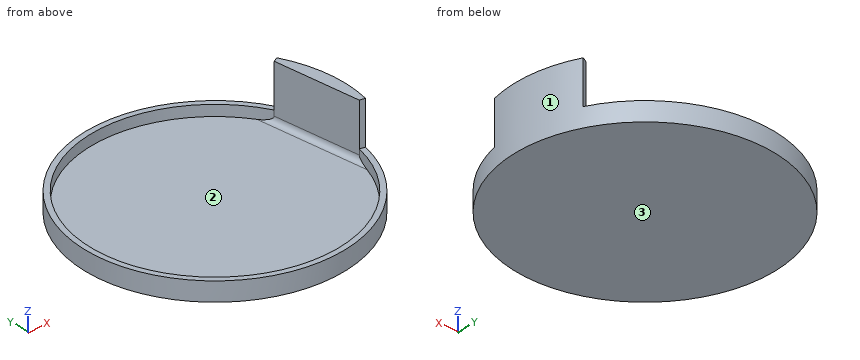
```python
from build123d import *

# Parameters (mm, degrees)
SKETCH1_R           = 48
BOSS_EXTRUDE1_DEPTH = 3
SKETCH2_R           = 48
SKETCH2_R_2         = 46
BOSS_EXTRUDE2_DEPTH = 4
BOSS_EXTRUDE3_DEPTH = 20
FILLET1_R           = 2


# Read off the part's stored shape, not the designer's step: Boss-Extrude3
with BuildPart() as part:
    # Sketch1 → Boss-Extrude1 (new body)
    with BuildSketch(Plane(origin=(0, 0, 0), x_dir=(0, 1, 0), z_dir=(0, 0, 1))):
        with Locations(Location((0, 0, 0), (0, 0, 270))):
            Circle(SKETCH1_R)
    extrude(amount=BOSS_EXTRUDE1_DEPTH)

    # Sketch2 → Boss-Extrude2 (add)
    with BuildSketch(Plane.XY.offset(3)):
        Circle(SKETCH2_R)
        Circle(SKETCH2_R_2, mode=Mode.SUBTRACT)
    extrude(amount=BOSS_EXTRUDE2_DEPTH)

    # Boss-Extrude3 outline → Boss-Extrude3 (add)
    with BuildSketch(Plane.XY.offset(3)):
        with BuildLine():
            ThreePointArc((46.862031324, -10.389899911), (47.589460087, 6.264446393), (42.576897618, 22.163208008))
            Line((42.576897618, 22.163208008), (40.802860217, 21.239741008))
            Line((40.802860217, 21.239741008), (44.909446686, -9.956987415))
            Line((44.909446686, -9.956987415), (46.862031324, -10.389899911))
        make_face()
    extrude(amount=BOSS_EXTRUDE3_DEPTH)

    # Fillet1
    fillet1_edges = [part.edges().sort_by_distance(p)[0] for p in [
        (42.856153452, 5.641376796, 3),
    ]]
    fillet(fillet1_edges, radius=FILLET1_R)


solid = part.part
```
Input: part model. Units: mm. Frame: model coordinates. Face numbers are marked on the shaded views. Round coordinates to 2 decimals unless told otherwise and drop trailing zeros. Write each loop counter-clockwise with the first axis right and the second up, starting at its lowest first coordinate (ties: lowest second). Pieces come first, ordered by that corner, then holes. Notation, with made-up numbers: (39.5, 1.25) -> (69.5, 1.25) arc R23 cw to (69.5, 25.25) -> close; hole circle Ø2 at (-10.5, 30). An arc over 180 degrees is marked (long way). Answer as CSV lines item,"result".
1. Section C-C (z = 11). Return the cut outline in (x, y).
Geometry says:
outline,"(40.8, 21.24) -> (44.91, -9.96) -> (46.86, -10.39) arc R48 ccw to (42.58, 22.16) -> close"
2. Section A-A (x = 0). Return the cut outline in (y, z).
Geometry says:
outline,"(-48, 0) -> (48, 0) -> (48, 7) -> (46, 7) -> (46, 3) -> (-46, 3) -> (-46, 7) -> (-48, 7) -> close"
3. Section B-B (y = -38). Return the cut outline in (x, z), plus the area to 3 significant figures.
Geometry says:
outline,"(-29.33, 0) -> (29.33, 0) -> (29.33, 7) -> (25.92, 7) -> (25.92, 3) -> (-25.92, 3) -> (-25.92, 7) -> (-29.33, 7) -> close"
area,"203 mm^2"
4. Contact query for flat-ended pins moving along their axis: P1, Ø10, axis at x = 36.5, y = -20.5, coming from the -Z side; P2, Ø3, axis at x = -13.5, y = 0.5, coming from the +Z side; P3, Ø12, axis at y = 27.5, z = 20, coming from the +X side; P4, Ø1, axis at x = -31, z = 6.5, coming from the -Y side. Output: stop coordinate, or through.
Geometry says:
P1,"stops at z = 0"
P2,"stops at z = 3"
P3,"stops at x = 42.92"
P4,"stops at y = -37.06"
5. Mould query, pull axis X, two halves, no side actions, for the marked faces 1, 2 and 3. Classes: +X half, -X half, draft (parallel to the pull), parting line (faces both ways), or undercut.
Geometry says:
face 1,"parting line"
face 2,"undercut"
face 3,"draft"
6. Ray query, L1, parallel to Y at x = 0, z = 5.5; L2, parallel to Z at x = 33.5, y = 13; L3, parallel to X at y = 0, z = 4.75. Return the intervals inside material, ascending. Write a range as [from, to].
Geometry says:
L1,"y = [-48, -46], [46, 48]"
L2,"z = [0, 3]"
L3,"x = [-48, -46], [43.58, 48]"
